Design review of the part built by this model. Coordinates are the model's own, in mm. Coordinates: 2 decimals unless noted, no trailing zeros. Loops run counter-clockwise (first coordinate to the right, second up) from the corner with the lowest first, then second, coordinate; pieces in that order, holes last. Notation, with made-up numbers: (-27, -22.75) -> (7, -22.75) arc R29 ccw to (7, 8.25) -> close; hole circle Ø8 at (82, 13). An arc over 180 degrees is marked (long way). Answer in a Markdown table with one row per item.
```python
from build123d import *

# Parameters (mm, degrees)
SKETCH1_W             = 36
SKETCH1_H             = 36
SKETCH1_R             = 1.5
BASE_SHAPE_DEPTH      = 1.65
ROUNDED_CORNERS_R     = 2
PINHEADER_HOLES_REACH = 27.509
SKETCH2_R             = 0.6


with BuildPart() as part:
    # Sketch1 → Base shape (new body)
    with BuildSketch(Plane(origin=(0, 0, 0), x_dir=(1, 0, 0), z_dir=(0, 1, 0))):
        Rectangle(SKETCH1_W, SKETCH1_H)
        with Locations(Location((-15.25, 15.25, 0), (0, 0, 270))):
            Circle(SKETCH1_R, mode=Mode.SUBTRACT)
        with Locations(Location((15.25, 15.25, 0), (0, 0, 90))):
            Circle(SKETCH1_R, mode=Mode.SUBTRACT)
        with Locations(Location((15.25, -15.25, 0), (0, 0, 270))):
            Circle(SKETCH1_R, mode=Mode.SUBTRACT)
        with Locations(Location((-15.25, -15.25, 0), (0, 0, 90))):
            Circle(SKETCH1_R, mode=Mode.SUBTRACT)
    extrude(amount=BASE_SHAPE_DEPTH)

    # Rounded corners
    rounded_corners_edges = [part.edges().sort_by_distance(p)[0] for p in [
        (18, 0.825, 18),
        (-18, 0.825, 18),
        (-18, 0.825, -18),
        (18, 0.825, -18),
    ]]
    fillet(rounded_corners_edges, radius=ROUNDED_CORNERS_R)

    # Sketch2 → Pinheader holes (cut, up to next)
    with BuildSketch(Plane(origin=(0, 1.65, 0), x_dir=(1, 0, 0), z_dir=(0, 1, 0)), mode=Mode.PRIVATE) as pinheader_holes_sk1:
        with Locations(Location((-5.11, 15.65, 0), (0, 0, 270))):
            Circle(SKETCH2_R)
    pinheader_holes_tool1 = extrude(pinheader_holes_sk1.sketch, amount=-PINHEADER_HOLES_REACH, mode=Mode.PRIVATE) & part.part
    # Sketch2 → Pinheader holes (cut, up to next)
    with BuildSketch(Plane(origin=(0, 1.65, 0), x_dir=(1, 0, 0), z_dir=(0, 1, 0)), mode=Mode.PRIVATE) as pinheader_holes_sk2:
        with Locations(Location((-7.65, 15.65, 0), (0, 0, 270))):
            Circle(SKETCH2_R)
    pinheader_holes_tool2 = extrude(pinheader_holes_sk2.sketch, amount=-PINHEADER_HOLES_REACH, mode=Mode.PRIVATE) & part.part
    # Sketch2 → Pinheader holes (cut, up to next)
    with BuildSketch(Plane(origin=(0, 1.65, 0), x_dir=(1, 0, 0), z_dir=(0, 1, 0)), mode=Mode.PRIVATE) as pinheader_holes_sk3:
        with Locations(Location((-2.57, 15.65, 0), (0, 0, 270))):
            Circle(SKETCH2_R)
    pinheader_holes_tool3 = extrude(pinheader_holes_sk3.sketch, amount=-PINHEADER_HOLES_REACH, mode=Mode.PRIVATE) & part.part
    # Sketch2 → Pinheader holes (cut, up to next)
    with BuildSketch(Plane(origin=(0, 1.65, 0), x_dir=(1, 0, 0), z_dir=(0, 1, 0)), mode=Mode.PRIVATE) as pinheader_holes_sk4:
        with Locations(Location((-5.11, 13.11, 0), (0, 0, 270))):
            Circle(SKETCH2_R)
    pinheader_holes_tool4 = extrude(pinheader_holes_sk4.sketch, amount=-PINHEADER_HOLES_REACH, mode=Mode.PRIVATE) & part.part
    # Sketch2 → Pinheader holes (cut, up to next)
    with BuildSketch(Plane(origin=(0, 1.65, 0), x_dir=(1, 0, 0), z_dir=(0, 1, 0)), mode=Mode.PRIVATE) as pinheader_holes_sk5:
        with Locations(Location((-2.57, 13.11, 0), (0, 0, 270))):
            Circle(SKETCH2_R)
    pinheader_holes_tool5 = extrude(pinheader_holes_sk5.sketch, amount=-PINHEADER_HOLES_REACH, mode=Mode.PRIVATE) & part.part
    # Sketch2 → Pinheader holes (cut, up to next)
    with BuildSketch(Plane(origin=(0, 1.65, 0), x_dir=(1, 0, 0), z_dir=(0, 1, 0)), mode=Mode.PRIVATE) as pinheader_holes_sk6:
        with Locations(Location((-7.65, 13.11, 0), (0, 0, 270))):
            Circle(SKETCH2_R)
    pinheader_holes_tool6 = extrude(pinheader_holes_sk6.sketch, amount=-PINHEADER_HOLES_REACH, mode=Mode.PRIVATE) & part.part
    # Sketch2 → Pinheader holes (cut, up to next)
    with BuildSketch(Plane(origin=(0, 1.65, 0), x_dir=(1, 0, 0), z_dir=(0, 1, 0)), mode=Mode.PRIVATE) as pinheader_holes_sk7:
        with Locations(Location((-2.57, -13.11, 0), (0, 0, 270))):
            Circle(SKETCH2_R)
    pinheader_holes_tool7 = extrude(pinheader_holes_sk7.sketch, amount=-PINHEADER_HOLES_REACH, mode=Mode.PRIVATE) & part.part
    # Sketch2 → Pinheader holes (cut, up to next)
    with BuildSketch(Plane(origin=(0, 1.65, 0), x_dir=(1, 0, 0), z_dir=(0, 1, 0)), mode=Mode.PRIVATE) as pinheader_holes_sk8:
        with Locations(Location((-2.57, -15.65, 0), (0, 0, 270))):
            Circle(SKETCH2_R)
    pinheader_holes_tool8 = extrude(pinheader_holes_sk8.sketch, amount=-PINHEADER_HOLES_REACH, mode=Mode.PRIVATE) & part.part
    # Sketch2 → Pinheader holes (cut, up to next)
    with BuildSketch(Plane(origin=(0, 1.65, 0), x_dir=(1, 0, 0), z_dir=(0, 1, 0)), mode=Mode.PRIVATE) as pinheader_holes_sk9:
        with Locations(Location((-5.11, -13.11, 0), (0, 0, 270))):
            Circle(SKETCH2_R)
    pinheader_holes_tool9 = extrude(pinheader_holes_sk9.sketch, amount=-PINHEADER_HOLES_REACH, mode=Mode.PRIVATE) & part.part
    # Sketch2 → Pinheader holes (cut, up to next)
    with BuildSketch(Plane(origin=(0, 1.65, 0), x_dir=(1, 0, 0), z_dir=(0, 1, 0)), mode=Mode.PRIVATE) as pinheader_holes_sk10:
        with Locations(Location((-5.11, -15.65, 0), (0, 0, 270))):
            Circle(SKETCH2_R)
    pinheader_holes_tool10 = extrude(pinheader_holes_sk10.sketch, amount=-PINHEADER_HOLES_REACH, mode=Mode.PRIVATE) & part.part
    # Sketch2 → Pinheader holes (cut, up to next)
    with BuildSketch(Plane(origin=(0, 1.65, 0), x_dir=(1, 0, 0), z_dir=(0, 1, 0)), mode=Mode.PRIVATE) as pinheader_holes_sk11:
        with Locations(Location((-7.65, -13.11, 0), (0, 0, 270))):
            Circle(SKETCH2_R)
    pinheader_holes_tool11 = extrude(pinheader_holes_sk11.sketch, amount=-PINHEADER_HOLES_REACH, mode=Mode.PRIVATE) & part.part
    # Sketch2 → Pinheader holes (cut, up to next)
    with BuildSketch(Plane(origin=(0, 1.65, 0), x_dir=(1, 0, 0), z_dir=(0, 1, 0)), mode=Mode.PRIVATE) as pinheader_holes_sk12:
        with Locations(Location((-7.65, -15.65, 0), (0, 0, 270))):
            Circle(SKETCH2_R)
    pinheader_holes_tool12 = extrude(pinheader_holes_sk12.sketch, amount=-PINHEADER_HOLES_REACH, mode=Mode.PRIVATE) & part.part
    add(pinheader_holes_tool1.solids().sort_by_distance((-5.11, 1.65, -15.65))[0], mode=Mode.SUBTRACT)
    add(pinheader_holes_tool2.solids().sort_by_distance((-7.65, 1.65, -15.65))[0], mode=Mode.SUBTRACT)
    add(pinheader_holes_tool3.solids().sort_by_distance((-2.57, 1.65, -15.65))[0], mode=Mode.SUBTRACT)
    add(pinheader_holes_tool4.solids().sort_by_distance((-5.11, 1.65, -13.11))[0], mode=Mode.SUBTRACT)
    add(pinheader_holes_tool5.solids().sort_by_distance((-2.57, 1.65, -13.11))[0], mode=Mode.SUBTRACT)
    add(pinheader_holes_tool6.solids().sort_by_distance((-7.65, 1.65, -13.11))[0], mode=Mode.SUBTRACT)
    add(pinheader_holes_tool7.solids().sort_by_distance((-2.57, 1.65, 13.11))[0], mode=Mode.SUBTRACT)
    add(pinheader_holes_tool8.solids().sort_by_distance((-2.57, 1.65, 15.65))[0], mode=Mode.SUBTRACT)
    add(pinheader_holes_tool9.solids().sort_by_distance((-5.11, 1.65, 13.11))[0], mode=Mode.SUBTRACT)
    add(pinheader_holes_tool10.solids().sort_by_distance((-5.11, 1.65, 15.65))[0], mode=Mode.SUBTRACT)
    add(pinheader_holes_tool11.solids().sort_by_distance((-7.65, 1.65, 13.11))[0], mode=Mode.SUBTRACT)
    add(pinheader_holes_tool12.solids().sort_by_distance((-7.65, 1.65, 15.65))[0], mode=Mode.SUBTRACT)


solid = part.part
```
(1) To check wall thickness, follow probe 1 along Z at (x, y) = (-5, 1); probe 2 along X at (y, z) = (0.4, -15.5); probe 3 along X at (y, z) = (0.55, 14). State the ranges of each line that lie inside material, in increasing order.
Evaluation:
| item | result |
|---|---|
| probe 1 | z = -18 to -16.24, -15.06 to -13.7, -12.52 to 12.52, 13.7 to 15.06, 16.24 to 18 |
| probe 2 | x = -18 to -16.73, -13.77 to -8.23, -7.07 to -5.69, -4.53 to -3.15, -1.99 to 13.77, 16.73 to 18 |
| probe 3 | x = -18 to -16.08, -14.42 to 14.42, 16.08 to 18 |
(2) Take a section at A-A on x = -5.11. Give the boundary of the cut face in (y, z), and give its area (3 significant figures).
Evaluation:
| item | result |
|---|---|
| outline | (0, -18) -> (1.65, -18) -> (1.65, -16.25) -> (0, -16.25) -> close; (0, -15.05) -> (1.65, -15.05) -> (1.65, -13.71) -> (0, -13.71) -> close; (0, -12.51) -> (1.65, -12.51) -> (1.65, 12.51) -> (0, 12.51) -> close; (0, 13.71) -> (1.65, 13.71) -> (1.65, 15.05) -> (0, 15.05) -> close; (0, 16.25) -> (1.65, 16.25) -> (1.65, 18) -> (0, 18) -> close |
| area | 51.5 mm² |
(3) Take a section at B-B on z = 14.5. Give the boundary of the cut face in (x, y).
Evaluation:
| item | result |
|---|---|
| outline | (-18, 0) -> (-16.55, 0) -> (-16.55, 1.65) -> (-18, 1.65) -> close; (-13.95, 0) -> (13.95, 0) -> (13.95, 1.65) -> (-13.95, 1.65) -> close; (16.55, 0) -> (18, 0) -> (18, 1.65) -> (16.55, 1.65) -> close |
(4) Take a section at C-C on y = 0.7. Count the separate pieces of the cut face and the enclosed holes in it, and give its area (3 significant figures).
Evaluation:
| item | result |
|---|---|
| separate pieces | 1 |
| enclosed holes | 16 |
| area | 1,250 mm² |
(5) Draft analysis for pull direction X (two halves, no side actions). For faces 1 (the cylindrical face through (17.4, 0.84, -17.43)), 2 (the cylindrical face through (-15.32, 0.81, 16.75)), 3 (the flat face through (0, 1.65, 0)), state which applies: pulls with the +X half, pulls with the -X half, needs draft (parallel to the pull), parting line crosses it, or undercut.
Evaluation:
| item | result |
|---|---|
| face 1 | pulls with the +X half |
| face 2 | undercut |
| face 3 | needs draft |
(6) For pin 1 (1.1 mm diameter, centred on x = -7.65, z = 15.65, fed in from -Y), flat-tipped, find the tip position at first contact; note if it passes through.
Evaluation:
| item | result |
|---|---|
| pin 1 | passes through |
